Here's the drawing with two shaded views (mm, measured from the low corner). I have some questions. Round coordinates to 2 decimals unless told otherwise and drop trailing zeros. Order: outer loops, then holes, each group sorted by start corner. A loop starts at its lowest first (then second) coordinate and runs counter-clockwise, first axis right, second up.
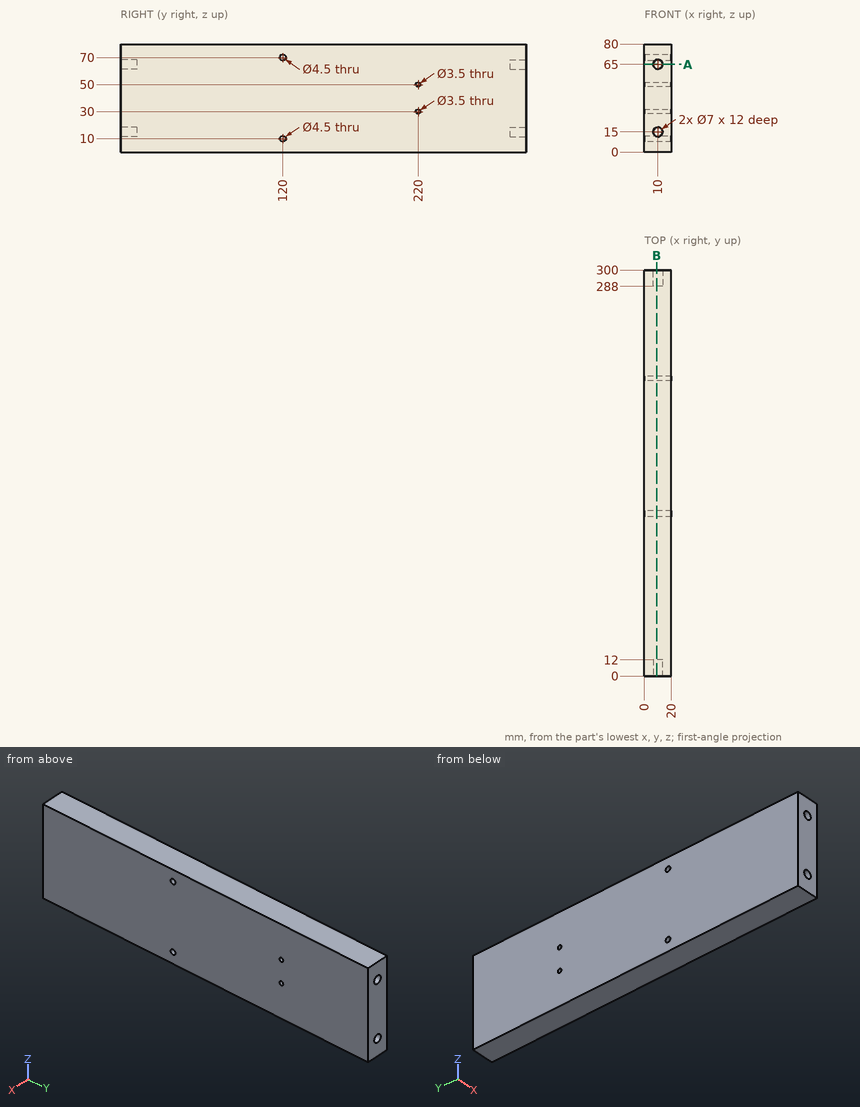
1. I'm going to push flat-ended pins straight in: P1, Ø6.5, axis at x = 10, z = 65, coming from the -Y side; P2, Ø2, axis at x = 11.5, z = 65.5, coming from the +Y side. Where does each tip first touch, or does it pass through?
Evaluation:
P1: stops at y = 12
P2: stops at y = 288
2. If we section it at A-A, the plane z = 65: Write out the boundary of the cut face in (x, y), and give its area (3 significant figures).
Evaluation:
outline: (0, 0) - (6.5, 0) - (6.5, 12) - (13.5, 12) - (13.5, 0) - (20, 0) - (20, 300) - (13.5, 300) - (13.5, 288) - (6.5, 288) - (6.5, 300) - (0, 300) - close
area: 5,830 mm2
3. I need wall thicknesses on probe 1 along Z at (x, y) = (7.5, 220); probe 2 along Z at (x, y) = (10, 295.5); probe 3 along Y at (x, z) = (10.5, 30). Which ranges of each line are inside material? Lowest first, please.
Evaluation:
probe 1: z = 0 to 28.25, 31.75 to 48.25, 51.75 to 80
probe 2: z = 0 to 11.5, 18.5 to 61.5, 68.5 to 80
probe 3: y = 0 to 218.25, 221.75 to 300
4. If we section it at B-B, the plane x = 9: Write out the boundary of the cut face in (y, z), and give its area (3 significant figures).
Evaluation:
outline: (0, 0) - (300, 0) - (300, 11.65) - (288, 11.65) - (288, 18.35) - (300, 18.35) - (300, 61.65) - (288, 61.65) - (288, 68.35) - (300, 68.35) - (300, 80) - (0, 80) - (0, 68.35) - (12, 68.35) - (12, 61.65) - (0, 61.65) - (0, 18.35) - (12, 18.35) - (12, 11.65) - (0, 11.65) - close; hole circle Ø4.5 at (120, 10); hole circle Ø4.5 at (120, 70); hole circle Ø3.5 at (220, 30); hole circle Ø3.5 at (220, 50)
area: 23,600 mm2
